Design review of the part shown in the three views and the two pictorial views. Dimensions are in mm from the part's minimum x, y and z. Give positions to 0.01 mm unless a question says otherwise; leave off trailing zeros. Loops run counter-clockwise (first coordinate to the right, second up) from the corner with the lowest first, then second, coordinate; pieces in that order, holes last.
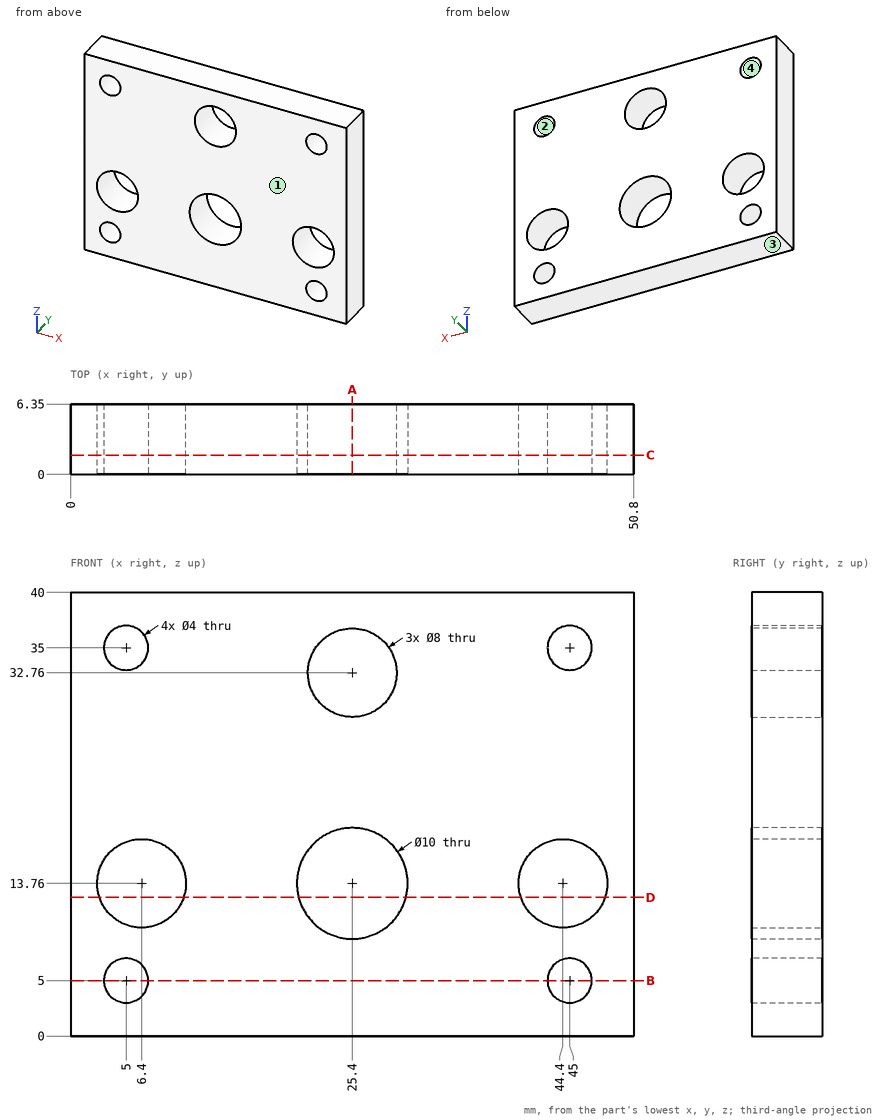
Q1. Consider section C-C on y = 1.75. Count the separate pieces of the cut face and the enclosed holes in it, plus the area to 3 significant figures.
Answers:
separate pieces: 1
enclosed holes: 8
area: 1,750 mm2
Q2. For probe 1 along X at (y, z) = (2.25, 5); probe 2 along Z at (x, y) = (25.5, 4.5); probe 3 along X at (y, z) = (3.5, 35) (1 decimal), list the stretches that pass through material, from the lowest coordinate up.
Answers:
probe 1: x = 0 to 3, 7 to 43, 47 to 50.8
probe 2: z = 0 to 8.76, 18.76 to 28.76, 36.76 to 40
probe 3: x = 0 to 3, 7 to 22.1, 28.7 to 43, 47 to 50.8
Q3. Consider section A-A on x = 25.4. Give the boundary of the cut face in (y, z).
Answers:
outline: (0, 0) - (6.35, 0) - (6.35, 8.76) - (0, 8.76) - close; (0, 18.76) - (6.35, 18.76) - (6.35, 28.76) - (0, 28.76) - close; (0, 36.76) - (6.35, 36.76) - (6.35, 40) - (0, 40) - close
Q4. Consider section B-B on z = 5. Give the boundary of the cut face in (x, y), plus the area to 3 significant figures.
Answers:
outline: (0, 0) - (3, 0) - (3, 6.35) - (0, 6.35) - close; (7, 0) - (43, 0) - (43, 6.35) - (7, 6.35) - close; (47, 0) - (50.8, 0) - (50.8, 6.35) - (47, 6.35) - close
area: 272 mm2
Q5. Mouldability with a two-part tool opening along Z and no side actions: class the marked faces 1, 2, 3 and 4 as +Z half, -Z half, draft (parallel to the pull), parting line (faces both ways), or undercut.
Answers:
face 1: draft
face 2: undercut
face 3: -Z half
face 4: undercut
Q6. Consider section D-D on z = 12.5. Give the boundary of the cut face in (x, y).
Answers:
outline: (0, 0) - (2.6, 0) - (2.6, 6.35) - (0, 6.35) - close; (10.2, 0) - (20.56, 0) - (20.56, 6.35) - (10.2, 6.35) - close; (30.24, 0) - (40.6, 0) - (40.6, 6.35) - (30.24, 6.35) - close; (48.2, 0) - (50.8, 0) - (50.8, 6.35) - (48.2, 6.35) - close
Q7. For pin 1 Ø5 at (x, z) = (25.4, 32.76) entering from -Y (1 decimal), flat-tipped, find the tip position at first contact; note if it passes through.
Answers:
pin 1: passes through
